For this review, take the finished solid that the model builds, in its own axes (mm). Coordinates: 2 decimals unless noted, no trailing zeros. Order: outer loops, then holes, each group sorted by start corner. A loop starts at its lowest first (then second) coordinate and runs counter-clockwise, first axis right, second up. Notation, with made-up numbers: (-6, -31.5) -> (26, -31.5) arc R24 cw to (26, -3.5) -> close; hole circle Ø9 at (50.25, -18). An arc over 180 degrees is marked (long way). Write item = value, one per line. Start each with the question number.
1) Consider section A-A on y = 30. Give the boundary of the cut face in (x, z).
2) Consider section D-D on y = 63. Give the boundary of the cut face in (x, z), and give its area (3 significant figures).
3) Draft analysis for pull direction Y (two halves, no side actions). For faces 1 (the face through (-1, 92, 2)), 2 (the face through (-17.95, 32.7, 0.99)), 3 (the face through (-15.867, 149.895, 0.986)), 4 (the face through (45, 45, 1)), state which applies: +Y half, -Y half, draft (parallel to the pull), parting line (faces both ways), or undercut.
4) Wall thickness on probe 1 along X at (y, z) = (153.8, 0.7); probe 2 along Y at (x, z) = (-15, 1.05); probe 3 along X at (y, z) = (28, 0.9): over which ranges is each line inside the solid? List them lowest first. Write a range as [from, to].
5) Consider section C-C on x = 15. Give the boundary of the cut face in (y, z).
6) Consider section B-B on z = 1.65. Give the boundary of the cut face in (x, y).
from build123d import *

# Parameters (mm, degrees)
CYLINDER_R             = 4
CYLINDER_DEPTH         = 10
CYLINDER001_R          = 4
CYLINDER001_DEPTH      = 10
CYLINDER002_R          = 4
CYLINDER002_DEPTH      = 10
CYLINDER003_R          = 4
CYLINDER003_DEPTH      = 10
BOX_W                  = 130
BOX_H                  = 130
BOX_DEPTH              = 2
FILLET_R               = 5
FILLET_PLACEMENT_ANGLE = 45


with BuildPart() as cylinder:
    # Cylinder → Cylinder (new body)
    with BuildSketch(Plane(origin=(15, 30, 0), x_dir=(1, 0, 0), z_dir=(0, 0, 1))):
        Circle(CYLINDER_R)
    extrude(amount=CYLINDER_DEPTH)


with BuildPart() as cylinder001:
    # Cylinder001 → Cylinder001 (new body)
    with BuildSketch(Plane(origin=(-15, 30, 0), x_dir=(1, 0, 0), z_dir=(0, 0, 1))):
        Circle(CYLINDER001_R)
    extrude(amount=CYLINDER001_DEPTH)


with BuildPart() as cylinder002:
    # Cylinder002 → Cylinder002 (new body)
    with BuildSketch(Plane(origin=(-15, 153.8, 0), x_dir=(1, 0, 0), z_dir=(0, 0, 1))):
        Circle(CYLINDER002_R)
    extrude(amount=CYLINDER002_DEPTH)


with BuildPart() as fusion:
    # Cylinder003 → Cylinder003 (new body)
    with BuildSketch(Plane(origin=(15, 153.8, 0), x_dir=(1, 0, 0), z_dir=(0, 0, 1))):
        Circle(CYLINDER003_R)
    extrude(amount=CYLINDER003_DEPTH)

    # Fusion: union Cylinder, Cylinder001, Cylinder002
    add(cylinder.part)
    add(cylinder001.part)
    add(cylinder002.part)


with BuildPart() as cut:
    # Box → Box (new body)
    with BuildSketch(Plane.XY):
        with Locations((65, 65)):
            Rectangle(BOX_W, BOX_H)
    extrude(amount=BOX_DEPTH)

    # Fillet
    fillet_edges = [cut.edges().sort_by_distance(p)[0] for p in [
        (0, 0, 1),
        (0, 130, 1),
        (130, 0, 1),
        (130, 130, 1),
    ]]
    fillet(fillet_edges, radius=FILLET_R)


with BuildPart() as cut_1:
    # Fillet placement: moved
    add(cut.part.rotate(Axis((0, 0, 0), (0, 0, 1)), FILLET_PLACEMENT_ANGLE))

    # Cut: cut Fusion
    add(fusion.part, mode=Mode.SUBTRACT)


solid = cut_1.part
Answer sheet:
q1.outline = (-30, 0) -> (-19, 0) -> (-19, 2) -> (-30, 2) -> close; (-11, 0) -> (11, 0) -> (11, 2) -> (-11, 2) -> close; (19, 0) -> (30, 0) -> (30, 2) -> (19, 2) -> close
q2.outline = (-63, 0) -> (63, 0) -> (63, 2) -> (-63, 2) -> close
q2.area = 252 mm2
q3.face_1 = draft
q3.face_2 = undercut
q3.face_3 = undercut
q3.face_4 = -Y half
q4.probe_1 = [-30.05, -19], [-11, 11], [19, 30.05]
q4.probe_2 = [15, 26], [34, 149.8], [157.8, 168.85]
q4.probe_3 = [-28, -18.46], [-11.54, 11.54], [18.46, 28]
q5.outline = (15, 0) -> (26, 0) -> (26, 2) -> (15, 2) -> close; (34, 0) -> (149.8, 0) -> (149.8, 2) -> (34, 2) -> close; (157.8, 0) -> (168.85, 0) -> (168.85, 2) -> (157.8, 2) -> close
q6.outline = (-88.39, 88.39) -> (-3.54, 3.54) arc R5 ccw to (3.54, 3.54) -> (88.39, 88.39) arc R5 ccw to (88.39, 95.46) -> (3.54, 180.31) arc R5 ccw to (-3.54, 180.31) -> (-88.39, 95.46) arc R5 ccw to start; hole circle Ø8 at (-15, 30); hole circle Ø8 at (-15, 153.8); hole circle Ø8 at (15, 30); hole circle Ø8 at (15, 153.8)
